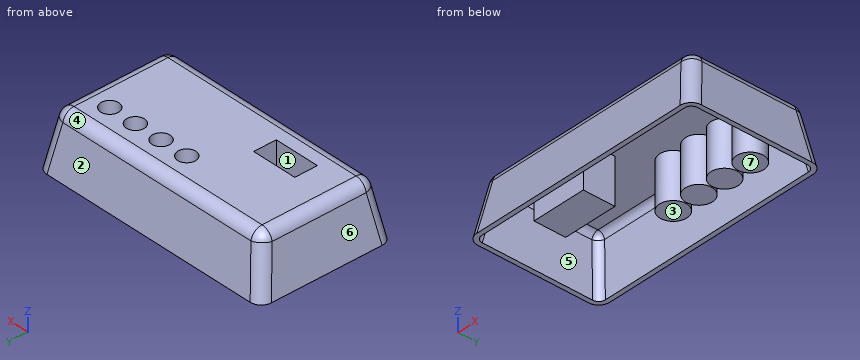
Solid Edge part; units mm, degrees
sketch "Sketch1" plane through (0, 0, 0) normal (0, 0, 1) x (1, 0, 0)
  line L0 (100, -50) -> (100, 50)
  line L1 (100, 50) -> (-100, 50)
  line L2 (-100, 50) -> (-100, -50)
  line L3 (-100, -50) -> (100, -50)
extrude "Protrusion1" add sketch "Sketch1" along normal blind 50
draft "Draft_1" angle 10 neutral plane through (0, 0, 50) normal (0, 0, 1) pull direction (0, 0, 1) face at (-68.6667, -50, 41.1667) face at (100, -34.3333, 41.1667) face at (68.6667, 50, 41.1667) face at (-100, 34.3333, 41.1667)
fillet "Round_1" radius 10 8 edges at (104.4082, -54.4082, 25) (104.4082, 54.4082, 25) (0, -50, 50) (100, 0, 50) (0, 50, 50) (-104.4082, -54.4082, 25) (-100, 0, 50) (-104.4082, 54.4082, 25)
sketch "Sketch2" plane through (0, 0, 50) normal (0, 0, 1) x (1, 0, 0)
  line L0 (-25.8045, -10.8045) -> (-65.8045, -10.8045)
  line L1 (-65.8045, -10.8045) -> (-65.8045, -30.8045)
  line L2 (-65.8045, -30.8045) -> (-25.8045, -30.8045)
  line L3 (-25.8045, -30.8045) -> (-25.8045, -10.8045)
  circle A0 centre (0, 25) radius 8
  circle A1 centre (25, 25) radius 8
  circle A2 centre (50, 25) radius 8
  circle A3 centre (75, 25) radius 8
extrude "Cutout_1" cut sketch "Sketch2" against normal blind 40
shell "Thin_Wall_1" thickness 4 removed faces 1 at (-74.7206, -38.0346, 0)
Could you check a few things on this model? Use its own coordinates, in mm. Face numbers are marked on the shaded views. A direction names the side the tool comes from. Coordinates: 2 decimals unless noted, no trailing zeros. Order: outer loops, then holes, each group sorted by start corner. A loop starts at its lowest first (then second) coordinate and runs counter-clockwise, first axis right, second up. Notation, with made-up numbers: (25, 84) - (52, 84) arc R16 ccw to (52, 94) - close; hole circle Ø1 at (54, 62). An arc over 180 degrees is marked (long way). Answer in a Markdown table with one row per item. Add a question column.
(1) If we section it at D-D, the plane y = -4.5: Please give me the cut outline in (x, z).
(2) I need wall thicknesses on L1, parallel to Y at x = 25, z = 21.5; L2, parallel to Y at x = -1.5, z = 8; L3, parallel to Y at x = 25, z = 29. Which ranges of each line are inside material? Lowest first, please.
(3) If we section it at A-A, the plane y = -16.5: Please give me the cut outline in (x, z).
(4) If we section it at C-C, the plane z = 15.5: State how many separate pieces and enclosed holes the cut face has, then the cut area to 3 significant figures.
(5) If we mould it in two halves opening along X, with no side actions, what happens to the marked faces 4, 5, 6 and 7? For each: released by +X, released by -X, zero draft, split by the parting line, or undercut.
(6) On a 3-axis mill with a long thin cutter (end or side, diameter ignored), from which of +Z, -Z, +X, -X, +Y, -Y can I reach the whole of each face in a straight line? I mean the marked faces 1, 2 and 3. Say none if no direction works.
(7) Will these pins go through, and if not, where does the flat tip stop? pin 1 (22.5 mm diameter, centred on y = -27, z = 29, fed in from -X); pin 2 (8 mm diameter, centred on x = 52, z = 8.5, fed in from -Y); pin 3 (6 mm diameter, centred on y = -7, z = 20, fed in from +X).
(8) If we section it at B-B, the plane x = 0: Please give me the cut outline in (y, z), then the cut area to 3 significant figures.
Results are:
| question | item | result |
|---|---|---|
| 1 | outline | (-108.82, 0) - (-104.75, 0) - (-97.52, 41.04) arc R6 cw to (-91.61, 46) - (91.61, 46) arc R6 cw to (97.52, 41.04) - (104.75, 0) - (108.82, 0) - (101.46, 41.74) arc R10 ccw to (91.61, 50) - (-91.61, 50) arc R10 ccw to (-101.46, 41.74) - close |
| 2 | L1 | y = -55.03 to -50.96, 13 to 17, 33 to 37, 50.96 to 55.03 |
| 2 | L2 | y = -57.41 to -53.34, 13.09 to 36.91, 53.34 to 57.41 |
| 2 | L3 | y = -53.7 to -49.64, 13 to 17, 33 to 37, 49.64 to 53.7 |
| 3 | outline | (-108.82, 0) - (-104.75, 0) - (-97.52, 41.04) arc R6 cw to (-91.61, 46) - (-69.8, 46) - (-69.8, 6) - (-21.8, 6) - (-21.8, 46) - (91.61, 46) arc R6 cw to (97.52, 41.04) - (104.75, 0) - (108.82, 0) - (101.46, 41.74) arc R10 ccw to (91.61, 50) - (-25.8, 50) - (-25.8, 10) - (-65.8, 10) - (-65.8, 50) - (-91.61, 50) arc R10 ccw to (-101.46, 41.74) - close |
| 4 | separate pieces | 6 |
| 4 | enclosed holes | 6 |
| 4 | area | 4,070 mm2 |
| 5 | face 4 | zero draft |
| 5 | face 5 | undercut |
| 5 | face 6 | released by -X |
| 5 | face 7 | undercut |
| 6 | face 1 | +Z |
| 6 | face 2 | +Z, +X, -X, +Y |
| 6 | face 3 | -Z |
| 7 | pin 1 | stops at x = -105.69 |
| 7 | pin 2 | stops at y = -58.02 |
| 7 | pin 3 | stops at x = 105.82 |
| 8 | outline | (-58.82, 0) - (-54.75, 0) - (-47.52, 41.04) arc R6 cw to (-41.61, 46) - (13, 46) - (13, 6) - (37, 6) - (37, 46) - (41.61, 46) arc R6 cw to (47.52, 41.04) - (54.75, 0) - (58.82, 0) - (51.46, 41.74) arc R10 ccw to (41.61, 50) - (33, 50) - (33, 10) - (17, 10) - (17, 50) - (-41.61, 50) arc R10 ccw to (-51.46, 41.74) - close |
| 8 | area | 1,080 mm2 |
